```python
from build123d import *

# Parameters (mm, degrees)
F0_W     = 128.114178
F0_H     = 110.934116
F0_R     = 39.096531
F1_DEPTH = 36.068
F2_R     = 50.357912
F2_R_2   = 39.406524
F3_DEPTH = 50.8


with BuildPart() as f1:
    # F0 (on Front) → F1 (new body)
    with BuildSketch(Plane.XZ):
        Rectangle(F0_W, F0_H)
        Circle(F0_R, mode=Mode.SUBTRACT)
    extrude(amount=-F1_DEPTH)

    # F2 (on Front) → F3 (join)
    with BuildSketch(Plane.XZ):
        Circle(F2_R)
        Circle(F2_R_2, mode=Mode.SUBTRACT)
    extrude(amount=F3_DEPTH)


solid = f1.part
```
Can you work these out from the model? Positions are in its coordinate system, mm. A direction names the side the tool comes from. Give positions to 0.01 mm unless a question says otherwise; leave off trailing zeros. Loops run counter-clockwise (first coordinate to the right, second up) from the corner with the lowest first, then second, coordinate; pieces in that order, holes last. Notation, with made-up numbers: M 11,9.25 L 30,9.25 A31 cw 30,45.25 Z; hole C -34.5,-33.5 d8. An arc over 180 degrees is marked long. One line per question, with ' | ' between items. Start each with the question number.
Q1. If we section it at D-D (x = -48): Please give me the cut outline in (y, z).
Q2. If we section it at C-C (y = 12): Please give me the cut outline in (x, z), plus the area to 3 significant figures.
Q3. If I drill on line 1 (Z direction, x = 0, y = 12); line 2 (Z direction, x = 0, y = -21); line 3 (Y direction, x = 39, z = -46.5), over which ranges is the centre line in solid material (lowest first)? Write a range as from..to.
Q4. If we section it at A-A (z = 0): Please give me the cut outline in (x, y).
Q5. If we section it at B-B (x = 0): Please give me the cut outline in (y, z), plus the area to 3 significant figures.
Q6. If we mould it in two halves opening along Z, with no side actions, what happens to faces 1 (the flat face through (-1, 18, -55.467)), 2 (the flat face through (-44, 0, 25)), 3 (the cylindrical face through (37.291, 17.782, 11.744)), 4 (the cylindrical face through (37.6, -25, 11.8))? For each: +Z half, -Z half, draft (parallel to the pull), parting line (faces both ways), or undercut.
Q7. For faces 5 (the cylindrical face through (48.03, -25.04, 15.13)), 6 (the flat face through (64.057, 18, -1)), which set-ups out of +Z, -Z, +X, -X, +Y, -Y let a thin tool reach every point of the face, with its end or its side?
Q8. For pin 1 Ø6 at (y, z) = (-31.5, -23.5) entering from +X; pin 2 Ø10 at (y, z) = (-39, 1) entering from +X; pin 3 Ø1.5 at (x, y) = (-9.5, -17) entering from +Z, each with a flat end and sliding along its axis, tell me the tip position at first contact or that it passes through.
Computed:
1) outline: M -50.8,-15.23 L 0,-15.23 L 0,-55.47 L 36.07,-55.47 L 36.07,55.47 L 0,55.47 L 0,15.23 L -50.8,15.23 Z
2) outline: M -64.06,-55.47 L 64.06,-55.47 L 64.06,55.47 L -64.06,55.47 Z; hole C 0,0 d78.19 | area: 9,410 mm²
3) line 1: z = -55.47..-39.1, 39.1..55.47 | line 2: z = -50.36..-39.41, 39.41..50.36 | line 3: y = 0..36.07
4) outline: M -64.06,0 L -50.36,0 L -50.36,-50.8 L -39.41,-50.8 L -39.41,0 L -39.1,0 L -39.1,36.07 L -64.06,36.07 Z; M 39.1,0 L 39.41,0 L 39.41,-50.8 L 50.36,-50.8 L 50.36,0 L 64.06,0 L 64.06,36.07 L 39.1,36.07 Z
5) outline: M -50.8,-50.36 L 0,-50.36 L 0,-55.47 L 36.07,-55.47 L 36.07,-39.1 L 0,-39.1 L 0,-39.41 L -50.8,-39.41 Z; M -50.8,39.41 L 0,39.41 L 0,39.1 L 36.07,39.1 L 36.07,55.47 L 0,55.47 L 0,50.36 L -50.8,50.36 Z | area: 2,290 mm²
6) face 1: -Z half | face 2: draft | face 3: undercut | face 4: undercut
7) face 5: -Y | face 6: +Z, -Z, +X, +Y, -Y
8) pin 1: stops at x = 46 | pin 2: stops at x = 50.36 | pin 3: stops at z = 49.59
